from build123d import *

# Parameters (mm, degrees)
SKETCH1_W                   = 48
SKETCH1_H                   = 76
BOSS_EXTRUDE1_DEPTH         = 10
SKETCH2_R                   = 5.5
SKETCH2_R_2                 = 2.5
CUT_EXTRUDE1_DEPTH          = 63.032249677
CUT_EXTRUDE2_DEPTH          = 40
FILLET1_R                   = 3.6
FILLET2_R                   = 2.5
M3_TAPPED_HOLE1_D           = 2.5
M3_TAPPED_HOLE1_CSINK_D     = 3.05
M3_TAPPED_HOLE1_CSINK_ANGLE = 90
CHAMFER1_SIZE               = 2
SKETCH6_R                   = 1.5
CUT_EXTRUDE3_DEPTH          = 10
BOSS_EXTRUDE2_DEPTH         = 6.8
CHAMFER2_SIZE               = 2
SKETCH8_W                   = 3
SKETCH8_H                   = 33.594295814
CUT_EXTRUDE4_DEPTH          = 5


with BuildPart() as part:
    # Sketch1 → Boss-Extrude1 (new body)
    with BuildSketch(Plane(origin=(0, 0, 0), x_dir=(1, 0, 0), z_dir=(0, 1, 0))):
        Rectangle(SKETCH1_W, SKETCH1_H)
    extrude(amount=BOSS_EXTRUDE1_DEPTH)

    # Sketch2 → Cut-Extrude1 (cut, through all)
    with BuildSketch(Plane.ZY.offset(24)):
        with Locations((-23, 10)):
            Circle(SKETCH2_R)
        with Locations((-7.531152857, 10)):
            Circle(SKETCH2_R)
        with Locations((11.608764346, 10)):
            Circle(SKETCH2_R_2)
        with Locations((22.5, 10)):
            Circle(SKETCH2_R_2)
    extrude(amount=-CUT_EXTRUDE1_DEPTH, mode=Mode.SUBTRACT)

    # Sketch3 → Cut-Extrude2 (cut)
    with BuildSketch(Plane.ZY.offset(24)):
        with BuildLine():
            Line((-30.575601228, 16.807330276), (-30.575601228, 2.210930276))
            Line((-30.575601228, 2.210930276), (-22.840601228, 2.210930276))
            ThreePointArc((-22.840601228, 2.210930276), (-19.946134653, 2.772905234), (-17.472254435, 4.377171194))
            ThreePointArc((-17.472254435, 4.377171194), (-15.105601228, 5.332165574), (-12.73894802, 4.377171194))
            ThreePointArc((-12.73894802, 4.377171194), (0.284776113, 8.838942121), (-10.941513582, 16.807330276))
            Line((-10.941513582, 16.807330276), (-30.575601228, 16.807330276))
        make_face()
        with BuildLine():
            Line((6.124741926, 18.195630094), (6.124741926, 4.592448506))
            Line((6.124741926, 4.592448506), (11.608764346, 4.592448506))
            ThreePointArc((11.608764346, 4.592448506), (13.597512463, 4.971432203), (15.307501103, 6.055261787))
            ThreePointArc((15.307501103, 6.055261787), (16.948477041, 6.705162469), (18.590697922, 6.058414065))
            ThreePointArc((18.590697922, 6.058414065), (26.266760255, 6.298858065), (26.068998857, 13.976138617))
            Line((26.068998857, 13.976138617), (6.124741926, 18.195630094))
        make_face()
    extrude(amount=-CUT_EXTRUDE2_DEPTH, mode=Mode.SUBTRACT)

    # Fillet1
    fillet1_edges = [part.edges().sort_by_distance(p)[0] for p in [
        (-4, 2.210930276, -30.575601228),
    ]]
    fillet(fillet1_edges, radius=FILLET1_R)

    # Fillet2
    fillet2_edges = [part.edges().sort_by_distance(p)[0] for p in [
        (-4, 4.592448506, 6.124741926),
    ]]
    fillet(fillet2_edges, radius=FILLET2_R)

    # M3 Tapped Hole1 (through all)
    with Locations(Plane(origin=(0, 10, 0), x_dir=(1, 0, 0), z_dir=(0, 1, 0))):
        with Locations((-20.75, 34.75), (20.75, 34.75), (20.75, -3.244475858), (-20.75, -3.244475858), (-20.75, -34.75), (20.75, -34.75)):
            CounterSinkHole(M3_TAPPED_HOLE1_D / 2, M3_TAPPED_HOLE1_CSINK_D / 2, counter_sink_angle=M3_TAPPED_HOLE1_CSINK_ANGLE)

    # Chamfer1
    chamfer1_edges = [part.edges().sort_by_distance(p)[0] for p in [
        (-24, 2.210930276, -24.908101228),
        (-24, 3.265345864, -29.52118564),
        (-24, 4.592448506, 10.116753136),
        (-24, 5.324681553, 6.856974973),
        (-24, 7.905465138, -30.575601228),
        (-24, 2.772905234, -19.946134653),
        (-24, 5.332165574, -15.105601228),
        (-24, 2.837756402, -4.320340718),
        (-24, 8.546224253, 6.124741926),
        (-24, 4.971432203, 13.597512463),
        (-24, 6.705162469, 16.948477041),
        (-24, 5.035673535, 24.459770758),
    ]]
    chamfer(chamfer1_edges, length=CHAMFER1_SIZE)


with BuildPart() as body_2:
    # Mirror1: mirrored copy
    add(part.part.mirror(Plane(origin=(0, 10, 0), x_dir=(0, 0, 1), z_dir=(0, -1, 0))))

    # Sketch6 → Cut-Extrude3 (cut)
    with BuildSketch(Plane(origin=(0, 20, 0), x_dir=(1, 0, 0), z_dir=(0, 1, 0))):
        with Locations(Location((20.75, 34.75, 0), (0, 0, 270))):
            Circle(SKETCH6_R)
        with Locations(Location((-20.75, 34.75, 0), (0, 0, 270))):
            Circle(SKETCH6_R)
        with Locations(Location((-20.75, -3.244475858, 0), (0, 0, 270))):
            Circle(SKETCH6_R)
        with Locations(Location((20.75, -3.244475858, 0), (0, 0, 270))):
            Circle(SKETCH6_R)
        with Locations(Location((20.75, -34.75, 0), (0, 0, 270))):
            Circle(SKETCH6_R)
        with Locations(Location((-20.75, -34.75, 0), (0, 0, 270))):
            Circle(SKETCH6_R)
    extrude(amount=-CUT_EXTRUDE3_DEPTH, mode=Mode.SUBTRACT)

    # Sketch7 → Boss-Extrude2 (add)
    with BuildSketch(Plane.ZY.offset(-16)):
        with BuildLine():
            Line((6.124741926, 12.907551494), (6.124741926, 10))
            Line((6.124741926, 10), (9.108764346, 10))
            ThreePointArc((9.108764346, 10), (11.608764346, 12.5), (14.108764346, 10))
            Line((14.108764346, 10), (20, 10))
            ThreePointArc((20, 10), (22.5, 12.5), (25, 10))
            Line((25, 10), (27.753321561, 10))
            ThreePointArc((27.753321561, 10), (24.459770758, 14.964326465), (18.590697922, 13.941585935))
            ThreePointArc((18.590697922, 13.941585935), (16.948477041, 13.294837531), (15.307501103, 13.944738213))
            ThreePointArc((15.307501103, 13.944738213), (13.597512463, 15.028567797), (11.608764346, 15.407551494))
            Line((11.608764346, 15.407551494), (8.624741926, 15.407551494))
            ThreePointArc((8.624741926, 15.407551494), (6.856974973, 14.675318447), (6.124741926, 12.907551494))
        make_face()
    extrude(amount=BOSS_EXTRUDE2_DEPTH)

    # Chamfer2
    chamfer2_edges = [body_2.edges().sort_by_distance(p)[0] for p in [
        (24, 15.5, -23),
        (24, 15.5, -7.531152857),
        (24, 12.5, 11.608764346),
        (24, 12.5, 22.5),
    ]]
    chamfer(chamfer2_edges, length=CHAMFER2_SIZE)

    # Sketch8 → Cut-Extrude4 (cut)
    with BuildSketch(Plane.XZ.offset(-10)):
        with Locations((16.34371358, -39.350695858)):
            Rectangle(SKETCH8_W, SKETCH8_H)
    extrude(amount=-CUT_EXTRUDE4_DEPTH, mode=Mode.SUBTRACT)


solid = body_2.part
Can you work these out from the model? Positions are in its coordinate system, mm. A direction names the side the tool comes from. Coordinates: 2 decimals unless noted, no trailing zeros. Loops run counter-clockwise (first coordinate to the right, second up) from the corner with the lowest first, then second, coordinate; pieces in that order, holes last. Notation, with made-up numbers: M -21,-35 L 25,-35 A15 cw 25,-22 Z; hole C 47,86 d10. An arc over 180 degrees is marked long. Return JSON: item names as keys, results as strings. Group by question number.
Item 1: Imagine slicing it at D-D (x = -10.5). Please give me the cut outline in (y, z) (1 decimal).
Item 2: On a 3-axis mill with a long thin cutter (end or side, diameter ignored), from which of +Z, -Z, +X, -X, +Y, -Y can I reach the whole of each face in a straight line? I mean faces 5 (the flat face through (6, 10, 3)), 6 (the flat face through (-7, 11, 6.125)), 7 (the flat face through (14.844, 12, -34)). Say none if no direction works.
Item 3: If I drill on L1, parallel to X at y = 14.75, z = 34.75; L2, parallel to Z at x = -11.5, y = 13.5; L3, parallel to Z at x = 21.5, y = 18.25, over which ranges is the centre line in solid material (lowest first)? Write a range as from..to.
Item 4: Imagine slicing it at B-B (x = 20.75). Give the number of separate pieces and of enclosed holes in the cut face, and give its area (3 significant figures).
Item 5: Thinking about a two-plate mould opening in X: for faces 1 (the conical face through (22.125, 15.624, -7.655)), 2 (the flat face through (-4, 12, -30.576)), 3 (the cylindrical face through (22.237, 15.082, 3.049)), 4 (the cylindrical face through (21.76, 15.08, 33.64)), which applies, released by +X, released by -X, zero draft, split by the parting line, or undercut?
Item 6: I'm going to push flat-ended pins straight in: pin 1 Ø1.8 at (x, z) = (-20.75, 34.75) entering from -Y; pin 2 Ø2.5 at (x, z) = (-12, 10.5) entering from -Y; pin 3 Ø5 at (x, z) = (4.5, -20.5) entering from -Y; pin 4 Ø4 at (y, z) = (12, -19.5) entering from -X. Where does each tip first touch, or does it pass through?
Item 7: Imagine slicing it at A-A (z = 34.75). Please give me the cut outline in (x, y) (3 decimals).
Item 8: Imagine slicing it at C-C (z = -34.75). Please give me the cut outline in (x, y) (3 decimals).
Verdict:
{
 "1": {"outline": "M 10,-38 L 20,-38 L 20,38 L 10,38 L 10,27.8 A5.4 cw 13.9,18.6 A2.4 ccw 13.9,15.3 A5.4 cw 15.4,11.6 L 15.4,8.6 A2.5 cw 12.9,6.1 L 10,6.1 L 10,0.4 A7.7 cw 15.6,-12.7 A3.4 ccw 15.6,-17.5 A7.7 cw 17.8,-22.8 L 17.8,-27 A3.6 cw 14.2,-30.6 L 10,-30.6 Z"},
 "2": {"face 5": "+Z, -Z, +X, -X, -Y", "face 6": "-X, -Y", "face 7": "-Z, -Y"},
 "3": {"L1": "x = -24..-22.25, -19.25..19.25, 22.25..24", "L2": "z = -38..-30.58, -0.45..6.2, 15.98..17.92, 26.45..38", "L3": "z = -38..-36.05, -33.45..1.95, 4.54..33.45, 36.05..38"},
 "4": {"separate pieces": "4", "enclosed holes": "0", "area": "555 mm^2"},
 "5": {"face 1": "released by +X", "face 2": "zero draft", "face 3": "undercut", "face 4": "undercut"},
 "6": {"pin 1": "passes through", "pin 2": "stops at y = 15.41", "pin 3": "stops at y = 16.09", "pin 4": "stops at x = 16"},
 "7": {"outline": "M -24,10 L -22.275,10 L -22.25,10.025 L -22.25,20 L -24,20 Z; M -19.25,10.025 L -19.225,10 L 19.225,10 L 19.25,10.025 L 19.25,20 L -19.25,20 Z; M 22.25,10.025 L 22.275,10 L 24,10 L 24,20 L 22.25,20 Z"},
 "8": {"outline": "M -24,10 L -22.275,10 L -22.25,10.025 L -22.25,20 L -24,20 Z; M -19.25,10.025 L -19.225,10 L 14.844,10 L 14.844,15 L 17.844,15 L 17.844,10 L 19.225,10 L 19.25,10.025 L 19.25,20 L -19.25,20 Z; M 22.25,10.025 L 22.275,10 L 24,10 L 24,20 L 22.25,20 Z"}
}
